Could you check a few things on this model? Use its own coordinates, in mm. A direction names the side the tool comes from. Round coordinates to 2 decimals unless told otherwise and drop trailing zeros. Write each loop counter-clockwise with the first axis right and the second up, starting at its lowest first coordinate (ties: lowest second). Pieces come first, ordered by that corner, then holes.
```python
from build123d import *

# Parameters (mm, degrees)
BOX011_W          = 10
BOX011_H          = 21
BOX011_DEPTH      = 12
CHAMFER001_SIZE   = 2
CYLINDER032_R     = 30
CYLINDER032_DEPTH = 10
CYLINDER031_R     = 30
CYLINDER031_DEPTH = 10
CYLINDER030_R     = 30
CYLINDER030_DEPTH = 10
CYLINDER028_R     = 30
CYLINDER028_DEPTH = 10
CYLINDER029_R     = 70
CYLINDER029_DEPTH = 10
CYLINDER027_R     = 70
CYLINDER027_DEPTH = 10
CYLINDER026_R     = 70
CYLINDER026_DEPTH = 10
CYLINDER025_R     = 70
CYLINDER025_DEPTH = 10
BOX008_W          = 10
BOX008_H          = 24
BOX008_DEPTH      = 15


with BuildPart() as chamfer001:
    # Box011 → Box011 (new body)
    with BuildSketch(Plane(origin=(2, 12, 9), x_dir=(1, 0, 0), z_dir=(0, 0, 1))):
        with Locations((5, 10.5)):
            Rectangle(BOX011_W, BOX011_H)
    extrude(amount=BOX011_DEPTH)

    # Chamfer001
    chamfer001_edges = [chamfer001.edges().sort_by_distance(p)[0] for p in [
        (7, 12, 9),
        (7, 12, 21),
        (7, 33, 9),
        (7, 33, 21),
    ]]
    chamfer(chamfer001_edges, length=CHAMFER001_SIZE)


with BuildPart() as chamfer001_1:
    # Chamfer001 placement: moved
    add(chamfer001.part.moved(Location((0, 135, 0))))


with BuildPart() as cylinder032:
    # Cylinder032 → Cylinder032 (new body)
    with BuildSketch(Plane(origin=(22, -27, 39.5), x_dir=(0, 0, -1), z_dir=(1, 0, 0))):
        Circle(CYLINDER032_R)
    extrude(amount=CYLINDER032_DEPTH)


with BuildPart() as cylinder031:
    # Cylinder031 → Cylinder031 (new body)
    with BuildSketch(Plane(origin=(22, -27, -24.5), x_dir=(0, 0, -1), z_dir=(1, 0, 0))):
        Circle(CYLINDER031_R)
    extrude(amount=CYLINDER031_DEPTH)


with BuildPart() as cylinder030:
    # Cylinder030 → Cylinder030 (new body)
    with BuildSketch(Plane(origin=(22, 27, -24.5), x_dir=(0, 0, -1), z_dir=(1, 0, 0))):
        Circle(CYLINDER030_R)
    extrude(amount=CYLINDER030_DEPTH)


with BuildPart() as cylinder028:
    # Cylinder028 → Cylinder028 (new body)
    with BuildSketch(Plane(origin=(22, 27, 39.5), x_dir=(0, 0, -1), z_dir=(1, 0, 0))):
        Circle(CYLINDER028_R)
    extrude(amount=CYLINDER028_DEPTH)


with BuildPart() as cylinder029:
    # Cylinder029 → Cylinder029 (new body)
    with BuildSketch(Plane(origin=(22, -58, 7.5), x_dir=(0, 0, -1), z_dir=(1, 0, 0))):
        Circle(CYLINDER029_R)
    extrude(amount=CYLINDER029_DEPTH)


with BuildPart() as cylinder027:
    # Cylinder027 → Cylinder027 (new body)
    with BuildSketch(Plane(origin=(22, 58, 7.5), x_dir=(0, 0, -1), z_dir=(1, 0, 0))):
        Circle(CYLINDER027_R)
    extrude(amount=CYLINDER027_DEPTH)


with BuildPart() as cylinder026:
    # Cylinder026 → Cylinder026 (new body)
    with BuildSketch(Plane(origin=(22, 0, 84.5), x_dir=(0, 0, -1), z_dir=(1, 0, 0))):
        Circle(CYLINDER026_R)
    extrude(amount=CYLINDER026_DEPTH)


with BuildPart() as cylinder025:
    # Cylinder025 → Cylinder025 (new body)
    with BuildSketch(Plane(origin=(22, 0, -69.5), x_dir=(0, 0, -1), z_dir=(1, 0, 0))):
        Circle(CYLINDER025_R)
    extrude(amount=CYLINDER025_DEPTH)


with BuildPart() as cut029:
    # Box008 → Box008 (new body)
    with BuildSketch(Plane(origin=(22, -12, 0), x_dir=(1, 0, 0), z_dir=(0, 0, 1))):
        with Locations((5, 12)):
            Rectangle(BOX008_W, BOX008_H)
    extrude(amount=BOX008_DEPTH)

    # Cut015: cut Cylinder025
    add(cylinder025.part, mode=Mode.SUBTRACT)

    # Cut016: cut Cylinder026
    add(cylinder026.part, mode=Mode.SUBTRACT)

    # Common004: intersect Cylinder027
    add(cylinder027.part, mode=Mode.INTERSECT)

    # Common005: intersect Cylinder029
    add(cylinder029.part, mode=Mode.INTERSECT)

    # Cut017: cut Cylinder028
    add(cylinder028.part, mode=Mode.SUBTRACT)

    # Cut018: cut Cylinder030
    add(cylinder030.part, mode=Mode.SUBTRACT)

    # Cut019: cut Cylinder031
    add(cylinder031.part, mode=Mode.SUBTRACT)

    # Cut020: cut Cylinder032
    add(cylinder032.part, mode=Mode.SUBTRACT)


with BuildPart() as cut029_1:
    # Cut020 placement: moved
    add(cut029.part.moved(Location((-20, 157.5, 7.5))))

    # Cut029: cut Chamfer001
    add(chamfer001_1.part, mode=Mode.SUBTRACT)


solid = cut029_1.part
```
Q1. Imagine slicing it at B-B, the plane z = 17.75. Write out the boundary of the cut face in (x, y), then the cut area to 3 significant figures.
Q2. If I drill on L1, parallel to Z at x = 9, y = 158.25; L2, parallel to Z at x = 6.25, y = 161.25; L3, parallel to Y at x = 3.5, z = 9.25, over which ranges is the centre line in solid material (lowest first)?
Q3. Imagine slicing it at D-D, the plane z = 21.75. Write out the boundary of the cut face in (x, y).
Q4. I'm going to push flat-ended pins straight in: pin 1 Ø5 at (x, y) = (9, 161) entering from +Z; pin 2 Ø1.5 at (x, z) = (5, 10.5) entering from -Y; pin 3 Ø6 at (x, y) = (7.5, 164.5) entering from -Z; pin 4 Ø1 at (x, y) = (5.5, 158.5) entering from -Z. Where does each tip first touch, or does it pass through?
Q5. We'd pull the mould along Z, two halves only. Please class faces 3 (the flat face through (7, 158, 9)), 4 (the flat face through (2, 158.3, 21.6)), 5 (the cylindrical face through (6.93, 146.821, 8.172)): pulls with the +Z half, pulls with the -Z half, needs draft (parallel to the pull), parting line crosses it, or undercut.
Q6. On a 3-axis mill with a long thin cutter (end or side, diameter ignored), from which of +Z, -Z, +X, -X, +Y, -Y can I reach the whole of each face in a straight line? I mean faces 1 (the flat face through (7, 167, 20)), 2 (the cylindrical face through (6.93, 146.79, 21.81)). Say none if no direction works.
Q7. Imagine slicing it at C-C, the plane y = 165. Write out the boundary of the cut face in (x, z), then the cut area to 3 significant figures.
Q8. Imagine slicing it at A-A, the plane x = 6.75. Write out the boundary of the cut face in (y, z).
Results found:
1. outline: (2, 145.55) - (12, 145.55) - (12, 147) - (2, 147) - close; (2, 168) - (12, 168) - (12, 169.45) - (2, 169.45) - close
1. area: 28.9 mm2
2. L1: z = 8 to 9, 21 to 22
2. L2: z = 7.9 to 9, 21 to 22.1
2. L3: y = 145.74 to 148.75, 166.25 to 169.26
3. outline: (2, 146.7) - (12, 146.7) - (12, 168.3) - (2, 168.3) - close
4. pin 1: stops at z = 22.26
4. pin 2: stops at y = 145.6
4. pin 3: stops at z = 7.5
4. pin 4: stops at z = 7.98
5. face 3: undercut
5. face 4: needs draft
5. face 5: pulls with the -Z half
6. face 1: +X, -X
6. face 2: +Z, +X, -X, -Y
7. outline: (2, 7.6) - (12, 7.6) - (12, 9) - (2, 9) - close; (2, 21) - (12, 21) - (12, 22.4) - (2, 22.4) - close
7. area: 28.1 mm2
8. outline: (145.77, 8.82) arc R30 cw to (147.81, 7.5) - (149.15, 7.5) arc R70 cw to (165.85, 7.5) - (167.19, 7.5) arc R30 cw to (169.23, 8.82) arc R70 ccw to (169.23, 21.18) arc R30 cw to (167.19, 22.5) - (165.85, 22.5) arc R70 cw to (149.15, 22.5) - (147.81, 22.5) arc R30 cw to (145.77, 21.18) arc R70 ccw to start; hole (147, 11) - (149, 9) - (166, 9) - (168, 11) - (168, 19) - (166, 21) - (149, 21) - (147, 19) - close
